The listing builds one solid part. Answer for the finished solid, in the listing's coordinates (mm). Face numbers are marked on the shaded views. A direction names the side the tool comes from. Coordinates: 2 decimals unless noted, no trailing zeros. Write each loop counter-clockwise with the first axis right and the second up, starting at its lowest first coordinate (ties: lowest second). Pieces come first, ordered by that corner, then holes. Notation, with made-up numbers: M 7.5,63 L 27.5,63 A26 ccw 27.5,82 Z; hole C -3.75,33 d1. An arc over 180 degrees is marked long. Answer as a JSON object with one key per item and string values. Group by question number.
Autodesk Fusion 360 part; units mm, degrees
sketch "Sketch1" plane through (0, 0, 0) normal (0, 0, 1) x (1, 0, 0)
  line L0 (-0.725, 2.115) -> (0.725, 2.115)
  line L1 (0.725, 2.115) -> (0.725, -2.115)
  line L2 (0.725, -2.115) -> (-0.725, -2.115)
  line L3 (-0.725, -2.115) -> (-0.725, 2.115)
  line L4 (-0.725, 2.115) -> (0.725, -2.115) construction
  line L5 (0.725, 2.115) -> (-0.725, -2.115) construction
  line L6 (-2.115, 0.675) -> (2.115, 0.675)
  line L7 (2.115, 0.675) -> (2.115, -0.675)
  line L8 (2.115, -0.675) -> (-2.115, -0.675)
  line L9 (-2.115, -0.675) -> (-2.115, 0.675)
  line L10 (-2.115, 0.675) -> (2.115, -0.675) construction
  line L11 (2.115, 0.675) -> (-2.115, -0.675) construction
  circle A0 centre (0, 0) radius 2.75
  dimension "d21" = 1.45
  dimension "d22" = 4.23
  dimension "d23" = 4.23
  dimension "d24" = 1.35
  dimension "d25" = 5.5
extrude "Extrude1" add sketch "Sketch1" against normal blind 3.7
chamfer "Chamfer1" distance 0.235 angle 65 4 edges at (-2.115, 0, -3.7) (2.115, 0, -3.7) (0, -2.115, -3.7) (0, 2.115, -3.7) measured on face at (-1.6186, -1.0735, -3.7) measured on face at (-1.6186, -1.0735, -3.7) measured on face at (-1.6186, -1.0735, -3.7) measured on face at (-1.6186, -1.0735, -3.7)
chamfer "Chamfer2" distance 0.0889 angle 80 8 edges at (0.725, 1.5125, -3.7) (1.5375, 0.675, -3.7) (1.5375, -0.675, -3.7) (0.725, -1.5125, -3.7) (-0.725, -1.5125, -3.7) (-1.5375, -0.675, -3.7) (-1.5375, 0.675, -3.7) (-0.725, 1.5125, -3.7) measured on face at (-1.0549, 1.725, -3.7) measured on face at (-1.0549, 1.725, -3.7) measured on face at (-1.0549, 1.725, -3.7) measured on face at (-1.0549, 1.725, -3.7) measured on face at (-1.0549, 1.725, -3.7) measured on face at (-1.0549, 1.725, -3.7) measured on face at (-1.0549, 1.725, -3.7) measured on face at (-1.0549, 1.725, -3.7)
equation "width = 5.5 mm"
equation "depth = 5.5 mm"
equation "cross_xy = 4.23 mm"
equation "gap_x = 1.35 mm"
equation "gap_y = 1.45 mm"
equation "height = 3.7 mm"
equation "d15 = chamfer_cross"
equation "d16 = chamfer_cross_angle"
equation "d17 = chamfer_gap"
equation "d18 = chamfer_gap_angle"
equation "d21 = gap_y"
equation "d22 = cross_xy"
equation "d23 = cross_xy"
equation "d24 = gap_x"
equation "d25 = width"
equation "chamfer_cross_angle = 65 deg"
equation "chamfer_cross = 0.235 mm"
equation "chamfer_gap_angle = 80 deg"
equation "chamfer_gap = 0.088857 mm"
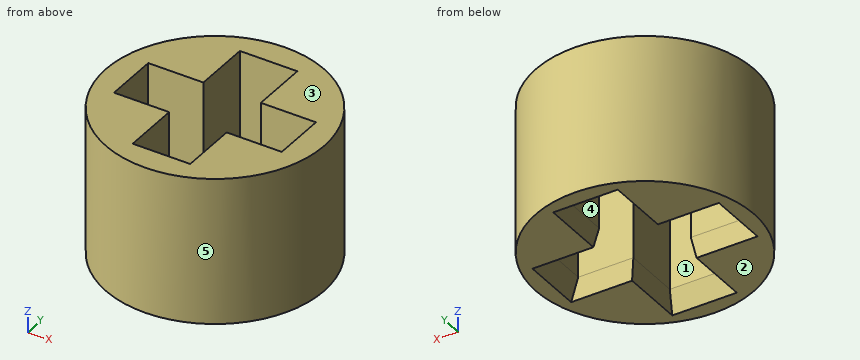
Item 1: A cutting plane is placed at D-D, the plane z = -3.4. Write down the section's boundary in (x, y), and give its area (3 significant figures).
Item 2: A tool of negligible diameter and unlimited length cuts with its end or side. For the marked faces 1 and 2, from which of +Z, -Z, +X, -X, +Y, -Y can it reach the whole face along a straight path? Write none if from no direction.
Item 3: Consider L1, parallel to X at y = 0.4, z = -2.75 (3 decimals); L2, parallel to Y at x = 0.95, z = -2.7 (3 decimals); L3, parallel to X at y = -0.85, z = -3.3. Determine where each line is inside the solid, lowest interval first. Write a range as from..to.
Item 4: A cutting plane is placed at A-A, the plane x = 0. Write down the section's boundary in (y, z) (3 decimals).
Item 5: Flat-ended cylindrical pins translate along their axes: pin 1 Ø0.7 at (x, z) = (-1, -1.5) entering from -Y; pin 2 Ø1.1 at (x, z) = (1.5, -1) entering from +Y; pin 3 Ø1.2 at (y, z) = (-1, -1.5) entering from +X. Find the tip coordinate at first contact, or state that the pin passes through.
Item 6: A cutting plane is placed at C-C, the plane z = -0.9. Write down the section's boundary in (x, y) (3 decimals), and give its area (3 significant figures).
Item 7: For a pull along Y with two mould halves and no side action, classify the marked faces 3, 4 and 5 as +Y half, -Y half, draft (parallel to the pull), parting line (faces both ways), or undercut.
Answer:
{
 "1": {"outline": "C 0,0 d5.5; hole M -2.21,-0.71 L -0.76,-0.71 L -0.76,-2.21 L 0.76,-2.21 L 0.76,-0.71 L 2.21,-0.71 L 2.21,0.71 L 0.76,0.71 L 0.76,2.21 L -0.76,2.21 L -0.76,0.71 L -2.21,0.71 Z", "area": "12.9 mm2"},
 "2": {"face 1": "+Z, -Z", "face 2": "-Z, +X, -X, +Y, -Y"},
 "3": {"L1": "-2.721..-2.115, 2.115..2.721", "L2": "-2.581..-0.675, 0.675..2.581", "L3": "-2.62..-0.74, 0.74..2.62"},
 "4": {"outline": "M -2.75,-3.7 L -2.35,-3.7 L -2.115,-3.196 L -2.115,0 L -2.75,0 Z; M 2.115,-3.196 L 2.35,-3.7 L 2.75,-3.7 L 2.75,0 L 2.115,0 Z"},
 "5": {"pin 1": "y = -2.67", "pin 2": "y = 2.58", "pin 3": "x = 2.72"},
 "6": {"outline": "C 0,0 d5.5; hole M -2.115,-0.675 L -0.725,-0.675 L -0.725,-2.115 L 0.725,-2.115 L 0.725,-0.675 L 2.115,-0.675 L 2.115,0.675 L 0.725,0.675 L 0.725,2.115 L -0.725,2.115 L -0.725,0.675 L -2.115,0.675 Z", "area": "13.9 mm2"},
 "7": {"face 3": "draft", "face 4": "undercut", "face 5": "parting line"}
}
